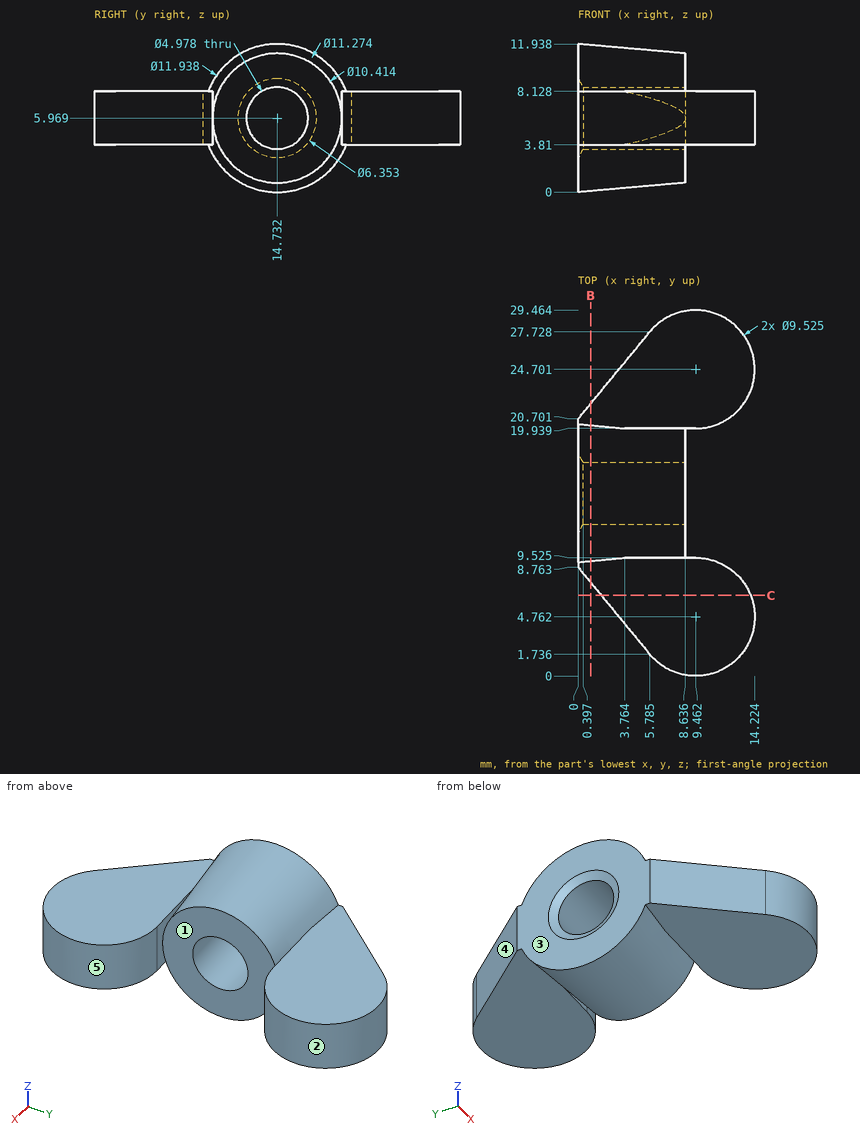
Job drawing, mm, ordinate dimensions from the low corner. One solid piece. A direction names the side the tool comes from. Coordinates: 2 decimals unless noted, no trailing zeros. Write each loop counter-clockwise with the first axis right and the second up, starting at its lowest first coordinate (ties: lowest second). Pieces come first, ordered by that corner, then holes. Notation, with made-up numbers: (68.5, 72.5) - (113.5, 72.5) arc R26 ccw to (113.5, 88.5) - close; hole circle Ø9 at (-3, 86). An arc over 180 degrees is marked (long way). Use a Markdown table: item, result. Add a question column.
Item 1: Band-saw the part on C-C, the plane y = 6.5. Give the cut face in (x, z) (1 decimal).
Item 2: Mould opens along Y. For the marked faces 3, 4 and 5 say: pulls with the +Y half, pulls with the -Y half, needs draft (parallel to the pull), parting line crosses it, or undercut.
Item 3: Flat gauge pins, fed straight in: pin 1 (2 mm diameter, centred on x = 6.5, z = 5.5, fed in from +Y); pin 2 (4 mm diameter, centred on x = 8.5, y = 5, fed in from -Z); pin 3 (4 mm diameter, centred on x = 10, y = 16.5, fed in from +Z). Where does each tip first touch, or does it go through?
Item 4: Band-saw the part on B-B, the plane x = 1. Give the cut face in (y, z) (1 decimal).
Item 5: Drill centre lines: L1, parallel to Y at x = 9.5, z = 7.25 (1 decimal); L2, parallel to Z at x = 4.75, y = 20; L3, parallel to Y at x = 12.75, z = 8 (1 decimal). Where is each one in solid material? Low to high. Write a range as from..to.
Item 6: 3-axis set-ups, long thin cutter, end or side, ignore diameter. For the marked faces 1 and 2: which of +Z, -Z, +X, -X, +Y, -Y reach the whole face in a straight line?
Numbers:
| question | item | result |
|---|---|---|
| 1 | outline | (1.9, 3.8) - (13.9, 3.8) - (13.9, 8.1) - (1.9, 8.1) - close |
| 2 | face 3 | needs draft |
| 2 | face 4 | pulls with the +Y half |
| 2 | face 5 | undercut |
| 3 | pin 1 | y = 29.04 |
| 3 | pin 2 | z = 3.81 |
| 3 | pin 3 | z = 11.17 |
| 4 | outline | (7.5, 3.8) - (9.3, 3.8) arc R5.9 ccw to (20.2, 3.8) - (21.9, 3.8) - (21.9, 8.1) - (20.2, 8.1) arc R5.9 ccw to (9.3, 8.1) - (7.5, 8.1) - close; hole circle Ø5 at (14.7, 6) |
| 5 | L1 | 0..9.5, 19.9..29.5 |
| 5 | L2 | 3.81..8.13 |
| 5 | L3 | 1.3..8.2, 21.3..28.1 |
| 6 | face 1 | +Z, -Z, +X |
| 6 | face 2 | +Z, -Z |
